Can you work these out from the model? Positions are in its coordinate system, mm. A direction names the side the tool comes from. Give positions to 0.01 mm unless a question says otherwise; leave off trailing zeros. Order: outer loops, then holes, each group sorted by start corner. A loop starts at its lowest first (then second) coordinate and runs counter-clockwise, first axis right, second up. Notation, with made-up numbers: (-11, 39) - (10, 39) arc R27 ccw to (10, 77) - close; hole circle Ø7 at (24, 21.25). An arc over 180 degrees is marked (long way). Return JSON: item names as keys, results as strings.
```python
from build123d import *

# Parameters (mm, degrees)
SKETCH_R     = 13.9
PAD_DEPTH    = 22.8
SKETCH001_R  = 13.7
PAD001_DEPTH = 12.9
FILLET_R     = 1
SKETCH002_W  = 1.549461
SKETCH002_H  = 7.151371
PAD002_DEPTH = 10.36


with BuildPart() as part:
    # Sketch → Pad (new body)
    with BuildSketch(Plane.XY):
        Circle(SKETCH_R)
    extrude(amount=-PAD_DEPTH)

    # Sketch001 → Pad001 (join)
    with BuildSketch(Plane.XY.offset(-22.8)):
        Circle(SKETCH001_R)
    extrude(amount=-PAD001_DEPTH)

    # Fillet
    fillet_edges = [part.edges().sort_by_distance(p)[0] for p in [
        (-13.7, 0, -35.7),
    ]]
    fillet(fillet_edges, radius=FILLET_R)

    # Sketch002 (on Face4 of Fillet) → Pad002 (join)
    with BuildSketch(Plane(origin=(0, 0, -35.7), x_dir=(1, 0, 0), z_dir=(0, 0, -1))):
        with Locations((-7.608272, -0.134424)):
            Rectangle(SKETCH002_W, SKETCH002_H)
    extrude(amount=PAD002_DEPTH)


solid = part.part
```
1. On a 3-axis mill with a long thin cutter (end or side, diameter ignored), from which of +Z, -Z, +X, -X, +Y, -Y can I reach the whole of each face in a straight line? I mean faces 1 (the face through (-8.383, 0, -41)), 2 (the face through (-10.097, 9.259, -28.667)), 3 (the face through (-8, -3.441, -41)). Say none if no direction works.
Checks:
{"face 1": "-Z, -X, +Y, -Y", "face 2": "-Z", "face 3": "-Z, +X, -X, -Y"}
2. Suppose I cut it at D-D (z = -30.5). List the corners of the cut face in (x, y) for me.
Checks:
{"outline": "circle Ø27.4 at (0, 0)"}
3. Suppose I cut it at C-C (z = -7.5). List the corners of the cut face in (x, y) for me.
Checks:
{"outline": "circle Ø27.8 at (0, 0)"}
4. For pin 1 Ø0.5 at (x, z) = (-7.5, -39.5) entering from -Y; pin 2 Ø8 at (y, z) = (-6.5, -37.5) entering from +X (3 decimals); pin 3 Ø1.5 at (x, z) = (2.5, -32) entering from -Y, each with a flat end and sliding along its axis, tell me the tip position at first contact or that it passes through.
Checks:
{"pin 1": "y = -3.44", "pin 2": "x = 13.235", "pin 3": "y = -13.59"}
5. Suppose I cut it at B-B (y = 0). List the corners of the cut face in (x, z) for me.
Checks:
{"outline": "(-13.9, -22.8) - (-13.7, -22.8) - (-13.7, -34.7) arc R1 ccw to (-12.7, -35.7) - (-8.38, -35.7) - (-8.38, -46.06) - (-6.83, -46.06) - (-6.83, -35.7) - (12.7, -35.7) arc R1 ccw to (13.7, -34.7) - (13.7, -22.8) - (13.9, -22.8) - (13.9, 0) - (-13.9, 0) - close"}
6. Suppose I cut it at A-A (x = 0). List the corners of the cut face in (y, z) for me.
Checks:
{"outline": "(-13.9, -22.8) - (-13.7, -22.8) - (-13.7, -34.7) arc R1 ccw to (-12.7, -35.7) - (12.7, -35.7) arc R1 ccw to (13.7, -34.7) - (13.7, -22.8) - (13.9, -22.8) - (13.9, 0) - (-13.9, 0) - close"}
7. If I drill on L1, parallel to Z at x = 6.25, y = 7.75; L2, parallel to Y at x = 1, z = -10; L3, parallel to Y at x = 5, z = -15, over which ranges is the centre line in solid material (lowest first)? Write a range as [from, to].
Checks:
{"L1": "[-35.7, 0]", "L2": "[-13.86, 13.86]", "L3": "[-12.97, 12.97]"}
